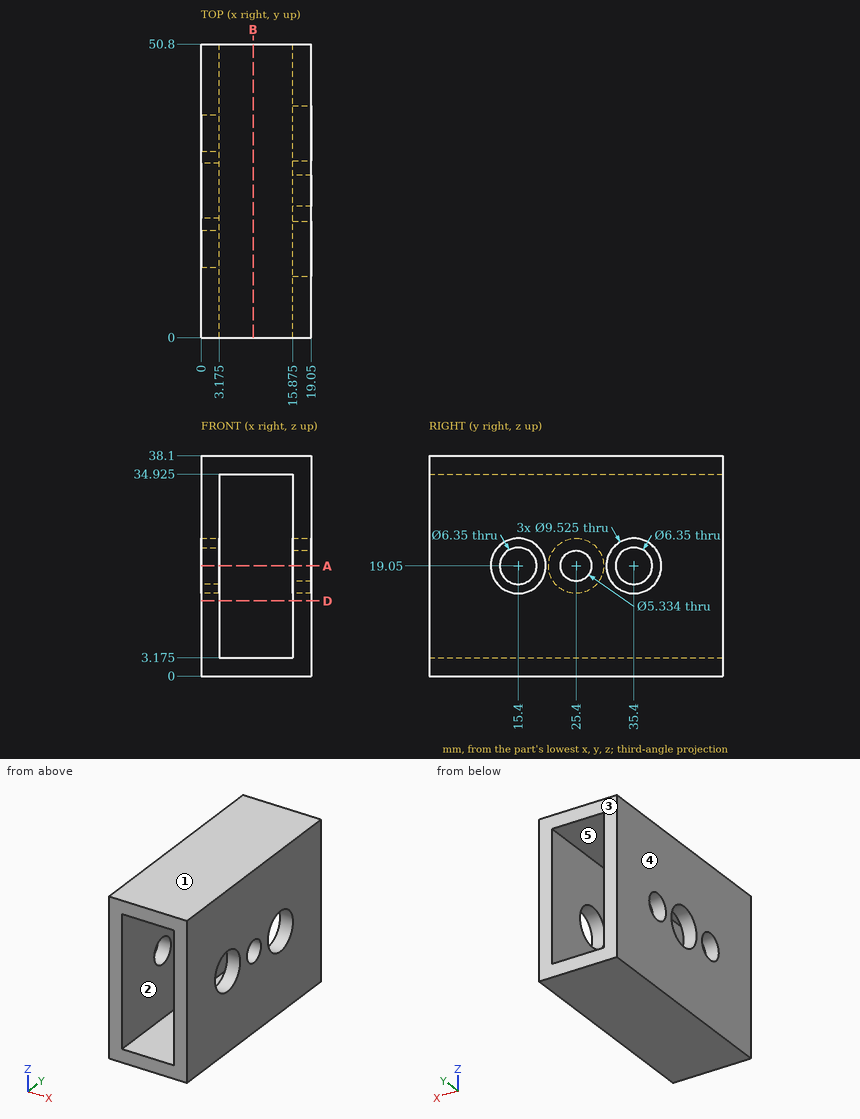
Input: dimensioned drawing with shaded views. Units: mm. Origin: part minimum x, y, z. A direction names the side the tool comes from. Round coordinates to 2 decimals unless told otherwise and drop trailing zeros. Write each loop counter-clockwise with the first axis right and the second up, starting at its lowest first coordinate (ties: lowest second). Pieces come first, ordered by that corner, then holes. Notation, with made-up numbers: (55.25, 49.5) -> (73.25, 49.5) arc R13 cw to (73.25, 55.5) -> close; hole circle Ø9 at (72, 53.5). An arc over 180 degrees is marked (long way). Use CSV: the item, a comma, the result in double quotes. Start each with the question number.
Q1. First-contact query: pin 1 Ø8.5 at (y, z) = (35.4, 19.05) entering from +X (3 decimals); pin 2 Ø5 at (y, z) = (35.4, 19.05) entering from +X. Flat tips, straight axial feed; report the tip coordinate or a pass-through.
Q2. Section A-A (z = 19.05). Give the number of separate pieces and of enclosed holes in the cut face, plus the area to 3 significant figures.
Q3. Pull-direction query (X, two-part tool) for the marked faces 3, 4 and 5; classes: pulls with the +X half, pulls with the -X half, needs draft (parallel to the pull), parting line crosses it, or undercut.
Q4. Section B-B (x = 9). Return loops of the section in (y, z) (3 decimals), plus the area to 3 significant figures.
Q5. Section D-D (z = 13). Return loops of the section in (x, y) (3 decimals).
Q6. Line query: L1, parallel to Y at x = 0.7, z = 19.05 (1 decimal); L2, parallel to Y at x = 17.75, z = 19.05; L3, parallel to Z at x = 8.25, y = 34 (3 decimals). Output: solid intervals per line, ascending.
Q7. Reachability of the marked faces 1 and 2 from +Z, -Z, +X, -X, +Y, -Y: full face, straight path, thin tool, end or side. Return the list, or none.
Result sheet:
1,pin 1,"x = 3.175"
1,pin 2,"through"
2,separate pieces,"8"
2,enclosed holes,"0"
2,area,"175 mm²"
3,face 3,"needs draft"
3,face 4,"pulls with the -X half"
3,face 5,"undercut"
4,outline,"(0, 0) -> (50.8, 0) -> (50.8, 3.175) -> (0, 3.175) -> close; (0, 34.925) -> (50.8, 34.925) -> (50.8, 38.1) -> (0, 38.1) -> close"
4,area,"323 mm²"
5,outline,"(0, 0) -> (3.175, 0) -> (3.175, 50.8) -> (0, 50.8) -> close; (15.875, 0) -> (19.05, 0) -> (19.05, 50.8) -> (15.875, 50.8) -> close"
6,L1,"0 to 12.2, 18.6 to 20.6, 30.2 to 32.2, 38.6 to 50.8"
6,L2,"0 to 10.64, 20.16 to 22.73, 28.07 to 30.64, 40.16 to 50.8"
6,L3,"0 to 3.175, 34.925 to 38.1"
7,face 1,"+Z, +X, -X, +Y, -Y"
7,face 2,"+Y, -Y"
